Here's how the part is built. I have some questions about the finished solid (model axes, mm). Round coordinates to 2 decimals unless told otherwise and drop trailing zeros. Loops run counter-clockwise (first coordinate to the right, second up) from the corner with the lowest first, then second, coordinate; pieces in that order, holes last. Notation, with made-up numbers: M -37,79.5 L 10,79.5 A29 cw 10,118.5 Z; hole C 50.5,-22.5 d1. An arc over 180 degrees is marked long. Answer as a JSON object with one key per item and string values.
from build123d import *

# Parameters (mm, degrees)
F0_W     = 170
F0_H     = 220
F0_H_2   = 82
F1_DEPTH = 1


with BuildPart() as f1:
    # F0 (on Top) → F1 (new body)
    with BuildSketch(Plane.XY):
        Polygon((36.485837, 841.869394), (-363.514163, 841.869394), (-363.514163, 361.869394), (-193.514163, 361.869394), (-73.514163, 361.869394), (36.485837, 361.869394), align=None)
        with Locations((-278.514163, 251.869394)):
            Rectangle(F0_W, F0_H)
        Polygon((-73.514163, 361.869394), (-193.514163, 361.869394), (-193.514163, 141.869394), (-193.514163, 59.869394), (-73.514163, 59.869394), align=None)
        with Locations((-278.514163, 100.869394)):
            Rectangle(F0_W, F0_H_2)
        Polygon((-193.514163, 59.869394), (-363.514163, 59.869394), (-363.514163, -285.130606), (-73.514163, -285.130606), (-73.514163, 59.869394), align=None)
    extrude(amount=F1_DEPTH)


solid = f1.part
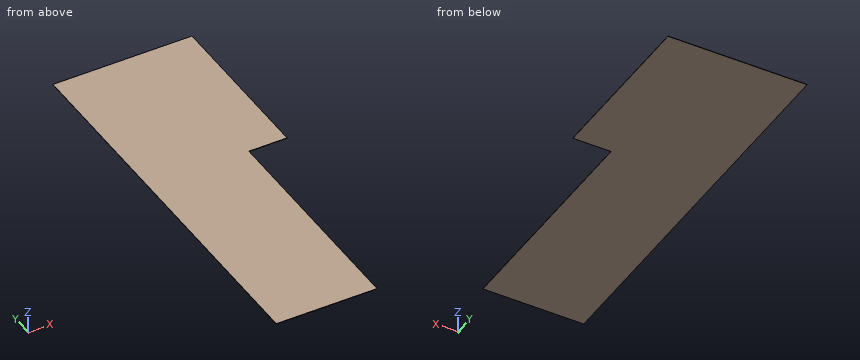
Item 1: I want a section at C-C, the plane y = -13. Please give me the cut outline in (x, z), then the cut area to 3 significant figures.
Resolved:
{"outline": "M -363.51,0 L -73.51,0 L -73.51,1 L -363.51,1 Z", "area": "290 mm²"}
Item 2: I want a section at B-B, the plane x = -62. Please give me the cut outline in (y, z), then the cut area to 3 significant figures.
Resolved:
{"outline": "M 361.87,0 L 841.87,0 L 841.87,1 L 361.87,1 Z", "area": "480 mm²"}
Item 3: Please list where these lines run through material, in increasing order: probe 1 along Y at (x, z) = (16, 0.9); probe 2 along X at (y, z) = (48, 0.75). Write a range as from..to.
Resolved:
{"probe 1": "361.87..841.87", "probe 2": "-363.51..-73.51"}
Item 4: I want a section at A-A, the plane z = 0.45. Please give me the cut outline in (x, y).
Resolved:
{"outline": "M -363.51,-285.13 L -73.51,-285.13 L -73.51,361.87 L 36.49,361.87 L 36.49,841.87 L -363.51,841.87 Z"}
Item 5: I'm going to push a flat-ended pin straight in: pin 1 Ø0.5 at (y, z) = (15, 0.5) entering from +X. Where does the tip first touch, or does it pass through?
Resolved:
{"pin 1": "x = -73.51"}
